Autodesk Inventor part; units mm, degrees
ref_plane "YZ Plane" through (0, 0, 0) normal (1, 0, 0) x (0, 1, 0)
ref_plane "XZ Plane" through (0, 0, 0) normal (0, 1, 0) x (-1, 0, 0)
ref_plane "XY Plane" through (0, 0, 0) normal (0, 0, 1) x (1, 0, 0)
sketch "Sketch1" plane through (0, 0, 0) normal (0, 0, 1) x (1, 0, 0)
  circle A0 centre (0, 0) radius 53.975 construction
  line L0 (-138.9624, -14.2875) -> (-138.9624, 14.2875) construction
  circle A1 centre (0, 0) radius 19.05
  line L1 (-181.8914, 0) -> (118.6116, 0)
  line L2 (0, -111.81) -> (0, 105.5438)
  line L3 (-3.175, -62.217) -> (-3.175, -64.2153)
  arc A2 (-52.8351, 11.0342) -> (-10.795, -52.8845) centre (0, 0) ccw
  arc A3 (-52.8351, 11.0342) -> (-55.4238, 19.7166) centre (-62.1589, 12.9814) ccw
  arc A4 (-3.175, -62.217) -> (-10.795, -52.8845) centre (-12.7, -62.217) ccw
  arc A5 (53.9096, -2.6565) -> (6.1993, 53.6178) centre (0, 0) ccw
  line L4 (1.9382, 56.6066) -> (-2.1738, 64.8531)
  arc A6 (3.4886, -70.5576) -> (67.6849, -20.231) centre (0, 0) ccw
  arc A7 (-7.6764, 67.8434) -> (-60.7093, 31.2417) centre (0, 0) ccw
  arc A8 (1.9382, 56.6066) -> (6.1993, 53.6178) centre (6.8266, 59.0442) ccw
  arc A9 (-2.1738, 64.8531) -> (-7.6764, 67.8434) centre (-7.0623, 62.4156) ccw
  line L5 (57.0769, -8.4682) -> (64.7759, -12.9132)
  arc A10 (53.9096, -2.6565) -> (57.0769, -8.4682) centre (60.2519, -2.969) ccw
  arc A11 (67.6849, -20.231) -> (64.7759, -12.9132) centre (61.6009, -18.4125) ccw
  arc A12 (-3.175, -64.2153) -> (3.4886, -70.5576) centre (3.175, -64.2153) ccw
  line L6 (-55.4238, 19.7166) -> (-59.5532, 23.846)
  arc A13 (-60.7093, 31.2417) -> (-59.5532, 23.846) centre (-55.063, 28.3361) ccw
  point P0 (-3.175, -53.8815)
  point P1 (-50.8, 57.9383)
  point P2 (-3.175, -53.8815)
  point P3 (-3.175, -70.4964)
  point P4 (-67.8823, 0)
  point P5 (3.3007, 53.874)
  point P6 (53.975, 0)
  point P7 (-3.8272, 68.169)
  point P8 (53.5878, -6.4538)
  point P9 (68.9605, -15.3293)
  point P10 (-3.175, -70.5724)
  point P11 (-62.7098, 27.0026)
  dimension "d0" = 107.95
  dimension "d10" = 38.1
  dimension "d14" = 3.175
  dimension "d15" = 9.525
  dimension "d79" = 30
  dimension "d80" = 6.35
  dimension "d89" = 6.35
  dimension "d97" = 70.6437
  dimension "d98" = 6.35
  dimension "d108" = 45
  dimension "d109" = 5.4625
  dimension "d110" = 8.89
extrude "Base" add sketch "Sketch1" along normal mid plane 6.35 contours L1 A5 A10 L5 A11 A6 A12 L2 A1 | A1 L2 L4 A8 A5 L1 | A1 L1 A2 A3 L6 A13 A7 A9 L4 L2 | L2 A12 L3 A4 A2 L1 A1
sketch "Sketch5" plane through (0, 0, -3.175) normal (0, 0, -1) x (-1, 0, 0)
  circle A0 centre (0, 0) radius 19.05
  arc A1 (60.7093, 31.2417) -> (7.6764, 67.8434) centre (0, 0) ccw
  circle A2 centre (0, 0) radius 53.975 construction
  line L0 (-53.2759, -12.7) -> (-58.4475, -17.8716) construction
  line L1 (-9.2461, -53.9826) -> (-14.6103, -59.3468) construction
  line L2 (91.9487, 0) -> (-94.6008, 0)
  line L3 (0, -99.577) -> (0, 103.505)
  arc A3 (-53.2759, -12.7) -> (-9.2461, -53.9826) centre (0, 0) ccw construction
  arc A4 (28.575, 46.7235) -> (-28.575, 46.7235) centre (0, 0) ccw construction
  arc A5 (-58.4475, -17.8716) -> (-14.6103, -59.3468) centre (0, 0) ccw construction
  arc A6 (28.575, 54.0275) -> (-28.575, 54.0275) centre (0, 0) ccw construction
  line L4 (-28.575, 46.7235) -> (-28.575, 54.0275) construction
  line L5 (28.575, 46.7235) -> (28.575, 54.0275) construction
  point P0 (40.1638, 60.9879)
  point P1 (-25.4, 51.9032)
  point P2 (25.4, 51.9032)
  point P3 (-54.2025, -18.1167)
  point P4 (-14.9213, -55.1677)
  dimension "d55" = 107.95
  dimension "d56" = 60.325
  dimension "d57" = 6.35
  dimension "d58" = 0.7937
  dimension "d59" = 57.15
  dimension "d60" = 6.35
  dimension "d61" = 0.7937
  dimension "d65" = 3.175
  dimension "d66" = 3.175
  dimension "d67" = 57.785
  dimension "d82" = 45
  dimension "d83" = 12.7
  dimension "d84" = 3.175
  dimension "d85" = 3.175
  dimension "d87" = 57.15
  dimension "d88" = 57.15
hole "Motor Stay Holes" at (25.4, 51.9032, -3.175) at (-25.4, 51.9032, -3.175) at (14.9213, -55.1677, -3.175) at (54.2025, -18.1167, -3.175) direction (0, 0, 1) diameter 3.175 end through all
sketch "Sketch6" plane through (0, 0, 3.175) normal (0, 0, 1) x (1, 0, 0)
  arc A0 (-3.175, -64.2153) -> (3.4886, -70.5576) centre (3.175, -64.2153) ccw
  arc A1 (-60.7093, 31.2417) -> (-59.5532, 23.846) centre (-55.063, 28.3361) ccw
hole "Standoff Holes to front plate" at (3.175, -64.2153, 3.175) at (-55.063, 28.3361, 3.175) direction (0, 0, -1) diameter 5.1054 end through all counterbore diameter 9.779 counterbore depth 1.5875
sketch "Sketch8" plane through (0, 0, -3.175) normal (0, 0, -1) x (-1, 0, 0)
  arc A0 (59.5532, 23.846) -> (60.7093, 31.2417) centre (55.063, 28.3361) ccw
  arc A1 (60.7093, 31.2417) -> (7.6764, 67.8434) centre (0, 0) ccw
  circle A2 centre (0, 0) radius 61.9263 construction
  arc A3 (10.795, -52.8845) -> (52.8351, 11.0342) centre (0, 0) ccw
  line L0 (0, 0) -> (43.7885, 43.7885) construction
  line L1 (94.4751, 0) -> (-104.0422, 0)
  line L2 (0, -111.81) -> (0, 105.5438)
  dimension "d119" = 45
hole "Standoff Holes to back plate" at (-43.7885, 43.7885, -3.175) direction (0, 0, 1) diameter 5.1054 end through all counterbore diameter 9.779 counterbore depth 1.5875
sketch "Sketch7" plane through (0, 0, 3.175) normal (0, 0, 1) x (1, 0, 0)
  arc A0 (3.4886, -70.5576) -> (67.6849, -20.231) centre (0, 0) ccw
  arc A1 (20.7648, -57.0509) -> (23.0757, -63.3999) centre (21.9203, -60.2254) ccw
  arc A2 (61.1475, -28.5135) -> (55.0241, -25.6581) centre (58.0858, -27.0858) ccw
  arc A3 (23.0757, -63.3999) -> (61.1475, -28.5135) centre (0, 0) ccw
  arc A4 (20.7648, -57.0509) -> (55.0241, -25.6581) centre (0, 0) ccw
  line L0 (58.0858, -27.0858) -> (0, 0) construction
  line L1 (0, 0) -> (21.9203, -60.2254) construction
  line L2 (-88.8322, 0) -> (103.1018, 0)
  line L3 (0, -110.4869) -> (0, 97.6056)
  dimension "d102" = 3.175
  dimension "d103" = 6.7564
  dimension "d104" = 25
  dimension "d105" = 20
extrude "Tensioning Slot" cut sketch "Sketch7" against normal through all
properties part number "motor plate"
Work out the finished part from the listing and answer in its coordinate system (mm). A direction names the side the tool comes from. Coordinates: 2 decimals unless noted, no trailing zeros. Write each loop counter-clockwise with the first axis right and the second up, starting at its lowest first coordinate (ties: lowest second). Pieces come first, ordered by that corner, then holes. Notation, with made-up numbers: M 6.25,24.5 L 27.25,24.5 A17 ccw 27.25,51.5 Z; hole C 5,-37 d4. An arc over 180 degrees is marked long. Answer as CSV lines item,"result". Start each with the question number.
Item 1: Flat-ended cylindrical pins translate along their axes: P1, Ø1.5, axis at y = 26, z = 1.5, coming from the +X side; P2, Ø8, axis at x = 3.18, y = -64.22, coming from the +Z side; P3, Ø3, axis at x = 3.5, y = -63.5, coming from the +Z side; P4, Ø1, axis at x = -40, y = 42.5, coming from the -Z side. Find the tip coordinate at first contact, or state that the pin passes through.
Item 2: Section B-B on x = 25 is taken. Write down the section's boundary in (y, z) (3 decimals), and give its area (3 significant figures).
Item 3: Section A-A on y = 0 is taken. Write down the section's boundary in (x, z) (3 decimals), and give its area (3 significant figures).
Item 4: Consider L1, parallel to Y at x = 4, z = -1.75; L2, parallel to X at y = 0, z = -1 (3 decimals); L3, parallel to X at y = -6.5, z = 0. Determine where each line is inside the solid, lowest interval first.
Item 5: A tool of negligible diameter and unlimited length cuts with its end or side. For faces 1 (the face through (-53.05, 15.77, -0.04)), 2 (the face through (-53, 26, 1.588)), 3 (the face through (40.77, -44.987, 0.044)), from which of +Z, -Z, +X, -X, +Y, -Y can it reach the whole face along a straight path? Write none if from no direction.
Item 6: Determine the mould class of faces 4 (the face through (-47.09, 40.18, -2.37)), 5 (the face through (45.3, -50, 0)), 6 (the face through (-4.5, 67.24, -0.04)), 7 (the face through (67.48, -16.01, -0.04)) for opening direction Y: released by +Y, released by -Y, zero draft, split by the parting line, or undercut.
Item 7: Section C-C on z = -0.5 is taken. Give the number of separate pieces and of enclosed holes in the cut face, and give its area (3 significant figures).
Checks:
1,P1,"stops at x = 47.7"
1,P2,"stops at z = 1.59"
1,P3,"passes through"
1,P4,"stops at z = -1.59"
2,outline,"M -66.072,-3.175 L -62.666,-3.175 L -62.666,3.175 L -66.072,3.175 Z; M -55.326,-3.175 L 47.836,-3.175 L 47.836,3.175 L -55.326,3.175 Z"
2,area,"677 mm²"
3,outline,"M -53.975,-3.175 L -19.05,-3.175 L -19.05,3.175 L -53.975,3.175 Z; M 19.05,-3.175 L 53.975,-3.175 L 53.975,3.175 L 19.05,3.175 Z"
3,area,"444 mm²"
4,L1,"y = -70.53 to -66.63, -61.8 to -18.63, 18.63 to 54.37"
4,L2,"x = -53.975 to -19.05, 19.05 to 53.975"
4,L3,"x = -53.58 to -17.91, 17.91 to 54.97"
5,face 1,"+Z, -Z, -X"
5,face 2,"+Z"
5,face 3,"+Z, -Z"
6,face 4,"undercut"
6,face 5,"undercut"
6,face 6,"released by +Y"
6,face 7,"split by the parting line"
7,separate pieces,"1"
7,enclosed holes,"8"
7,area,"10,100 mm²"
